from build123d import *

# Parameters (mm, degrees)
SKETCH1_R           = 2.35
BOSS_EXTRUDE1_DEPTH = 7
SKETCH2_R           = 2.75
BOSS_EXTRUDE2_DEPTH = 1.5


with BuildPart() as part:
    # Sketch1 → Boss-Extrude1 (new body)
    with BuildSketch(Plane(origin=(0, 0, 0), x_dir=(0, 0, -1), z_dir=(1, 0, 0))):
        Circle(SKETCH1_R)
    extrude(amount=BOSS_EXTRUDE1_DEPTH)

    # Sketch2 → Boss-Extrude2 (add)
    with BuildSketch(Plane(origin=(7, 0, 0), x_dir=(0, 0, -1), z_dir=(1, 0, 0))):
        Circle(SKETCH2_R)
    extrude(amount=BOSS_EXTRUDE2_DEPTH)

    # Sketch15 → Revolve1 (revolve)
    with BuildSketch(Plane.XY):
        with BuildLine():
            Line((0, 2.35), (0, -2.35))
            ThreePointArc((0, -2.35), (-2.35, 0), (0, 2.35))
        make_face()
    revolve(axis=Axis((0, 2.35, 0), (0, -1, 0)))


solid = part.part
Work out the finished part from the listing and answer in its coordinate system (mm). A direction names the side the tool comes from. Give positions to 0.01 mm unless a question says otherwise; leave off trailing zeros. Write each loop counter-clockwise with the first axis right and the second up, starting at its lowest first coordinate (ties: lowest second). Pieces come first, ordered by that corner, then holes. Notation, with made-up numbers: (69, -21) - (121, -21) arc R23 ccw to (121, -13) - close; hole circle Ø6 at (4, 77). An arc over 180 degrees is marked (long way). One line per item, written item: value. Start each with the question number.
1. Find section A-A (z = 0). Write down the section's boundary in (x, y), then the cut area to 3 significant figures.
2. Given pin 1 (1 mm diameter, centred on x = 4, y = 1.5, fed in from +Z); pin 2 (3 mm diameter, centred on x = 1, y = 1, fed in from +Z); pin 3 (3 mm diameter, centred on x = -1, z = 1.5, fed in from +Y), each flat-ended and moving along its own axis, determine where each tip first touches the part or whether it passes through.
3. For faces 1 (the flat face through (8.5, 0, 0)), 2 (the cylindrical face through (3.451, -2.294, 0.509)), determine the directions among +Z, -Z, +X, -X, +Y, -Y from which every point of the face is accessible in a straight line to the end or side of a thin tool.
4. Find section D-D (x = -0.5). Write down the section's boundary in (y, z), then the cut area to 3 significant figures.
5. Consider probe 1 along Y at (x, z) = (4, -0.1); probe 2 along X at (y, z) = (-2.25, -0.9); probe 3 along X at (y, z) = (0.6, 0.4). Determine where each line is inside the solid, lowest interval first.
6. Find section C-C (x = 6). Write down the section's boundary in (y, z).
Geometry results:
1. outline: (0, -2.35) - (7, -2.35) - (7, -2.75) - (8.5, -2.75) - (8.5, 2.75) - (7, 2.75) - (7, 2.35) - (0, 2.35) arc R2.35 ccw to start
1. area: 49.8 mm2
2. pin 1: z = 2.13
2. pin 2: z = 2.35
2. pin 3: y = 2.33
3. face 1: +Z, -Z, +X, +Y, -Y
3. face 2: -X
4. outline: circle Ø4.59 at (0, 0)
4. area: 16.6 mm2
5. probe 1: -2.35 to 2.35
5. probe 2: 7 to 8.5
5. probe 3: -2.24 to 8.5
6. outline: circle Ø4.7 at (0, 0)
